Geometry check sheet. Reference: the model listing, model coordinates, mm. Face numbers are marked on the shaded views. Round coordinates to 2 decimals unless told otherwise and drop trailing zeros. Order: outer loops, then holes, each group sorted by start corner. A loop starts at its lowest first (then second) coordinate and runs counter-clockwise, first axis right, second up.
(1) Go/stop test with flat-tipped pins: pin 1 (10 mm diameter, centred on x = 27, z = -23, fed in from +Y); pin 2 (3.5 mm diameter, centred on x = 101, z = -11, fed in from -Y). Record where each tip stops, or that it passes through.
(2) Sectioned sample at C-C (z = -69). Record the boundary of the cut face in (x, y).
(3) Material ranges on line 1 along X through (y, z) = (3.5, -23); line 2 along Z through (x, y) = (-3.5, 8.05); line 3 along Z through (x, y) = (99.5, 1.3), recorded low to high.
(4) Sectioned sample at D-D (x = 70.5). Record the boundary of the cut face in (y, z).
(5) Sectioned sample at A-A (y = 3.75). Give the number of separate pieces and of enclosed holes in the cut face, plus the area to 3 significant figures.
(6) Sectioned sample at B-B (z = -53). Record the boundary of the cut face in (x, y).
(7) Release check for a two-part mould opening along X. For the marked faces 1, 2 and 3 record: +X half, -X half, draft (parallel to the pull), parting line (faces both ways), or undercut.
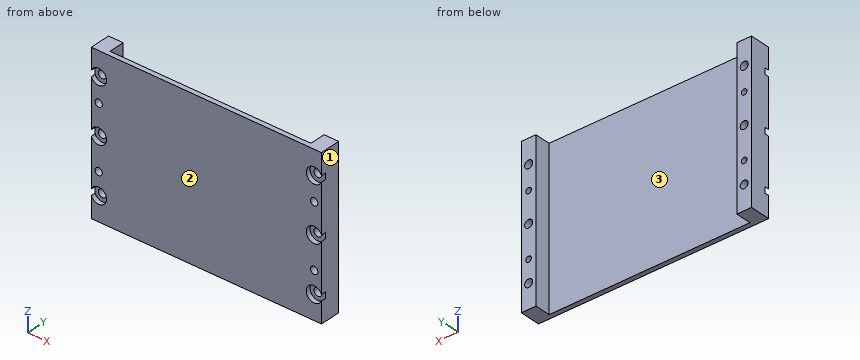
from build123d import *

# Parameters (mm, degrees)
SKETCH1_W                                      = 96
SKETCH1_H                                      = 75
BOSS_EXTRUDE1_DEPTH                            = 2.3
SKETCH2_W                                      = 7
SKETCH2_H                                      = 75
BOSS_EXTRUDE2_DEPTH                            = 7.5
BOSS_EXTRUDE2_DEPTH_BACK                       = 2.3
BOSS_EXTRUDE3_REACH                            = 9.5
SKETCH3_W                                      = 7
SKETCH3_H                                      = 75
BOSS_EXTRUDE3_DIRECTION_2_REACH                = 4.3
F_6_32_TAPPED_HOLE1_D                          = 2.7051
F_6_32_TAPPED_HOLE1_CBORE_D                    = 3.5052
F_6_32_TAPPED_HOLE1_CBORE_DEPTH                = 7.01
CBORE_FOR_6_BUTTON_HEAD_CAP_SCREW1_D           = 3.7973
CBORE_FOR_6_BUTTON_HEAD_CAP_SCREW1_CBORE_D     = 7.54126
CBORE_FOR_6_BUTTON_HEAD_CAP_SCREW1_CBORE_DEPTH = 2.1541994


with BuildPart() as part:
    # Sketch1 → Boss-Extrude1 (new body)
    with BuildSketch(Plane(origin=(0, 0, 0), x_dir=(1, 0, 0), z_dir=(0, 1, 0))):
        with Locations((48, 37.5)):
            Rectangle(SKETCH1_W, SKETCH1_H)
    extrude(amount=BOSS_EXTRUDE1_DEPTH)

    # Sketch2 → Boss-Extrude2 (add, two sides)
    with BuildSketch(Plane(origin=(0, 2.3, 0), x_dir=(1, 0, 0), z_dir=(0, 1, 0))) as boss_extrude2_sk:
        with Locations((-3.5, 37.5)):
            Rectangle(SKETCH2_W, SKETCH2_H)
    extrude(amount=BOSS_EXTRUDE2_DEPTH)
    extrude(boss_extrude2_sk.sketch, amount=-BOSS_EXTRUDE2_DEPTH_BACK)

    # Boss-Extrude3: up to this face of the body (flat: up to its plane)
    boss_extrude3_end = Plane(part.part.faces().sort_by_distance((-3.5, 9.8, -37.5))[0])
    # Sketch3 → Boss-Extrude3 (add, up to the picked face)
    with BuildSketch(Plane(origin=(0, 2.3, 0), x_dir=(1, 0, 0), z_dir=(0, 1, 0)), mode=Mode.PRIVATE) as boss_extrude3_sk1:
        with Locations((99.5, 37.5)):
            Rectangle(SKETCH3_W, SKETCH3_H)
    boss_extrude3_tool1 = split(extrude(boss_extrude3_sk1.sketch, amount=BOSS_EXTRUDE3_REACH, mode=Mode.PRIVATE), bisect_by=boss_extrude3_end, keep=Keep.BOTH, mode=Mode.PRIVATE)
    add(boss_extrude3_tool1.solids().sort_by_distance((99.5, 2.3, -37.5))[0])

    # Boss-Extrude3 direction 2: up to this face of the body (flat: up to its plane)
    boss_extrude3_direction_2_end = Plane(part.part.faces().sort_by_distance((44.5, 0, -37.5))[0])
    # Sketch3 → Boss-Extrude3 direction 2 (add, up to the picked face)
    with BuildSketch(Plane(origin=(0, 2.3, 0), x_dir=(1, 0, 0), z_dir=(0, 1, 0)), mode=Mode.PRIVATE) as boss_extrude3_direction_2_sk1:
        with Locations((99.5, 37.5)):
            Rectangle(SKETCH3_W, SKETCH3_H)
    boss_extrude3_direction_2_tool1 = split(extrude(boss_extrude3_direction_2_sk1.sketch, amount=-BOSS_EXTRUDE3_DIRECTION_2_REACH, mode=Mode.PRIVATE), bisect_by=boss_extrude3_direction_2_end, keep=Keep.BOTH, mode=Mode.PRIVATE)
    add(boss_extrude3_direction_2_tool1.solids().sort_by_distance((99.5, 2.3, -37.5))[0])

    # #6-32 Tapped Hole1 (through all)
    with Locations(Plane(origin=(0, 0, 0), x_dir=(-1, 0, 0), z_dir=(0, -1, 0))):
        with Locations((-99.5, 23), (-99.5, 53), (3.5, 23), (3.5, 53)):
            CounterBoreHole(F_6_32_TAPPED_HOLE1_D / 2, F_6_32_TAPPED_HOLE1_CBORE_D / 2, F_6_32_TAPPED_HOLE1_CBORE_DEPTH)

    # CBORE for #6 Button Head Cap Screw1 (through all)
    with Locations(Plane(origin=(0, 0, 0), x_dir=(-1, 0, 0), z_dir=(0, -1, 0))):
        with Locations((-99.5, 63.5), (-99.5, 37.5), (-99.5, 11.5), (3.5, 11.5), (3.5, 37.5), (3.5, 63.5)):
            CounterBoreHole(CBORE_FOR_6_BUTTON_HEAD_CAP_SCREW1_D / 2, CBORE_FOR_6_BUTTON_HEAD_CAP_SCREW1_CBORE_D / 2, CBORE_FOR_6_BUTTON_HEAD_CAP_SCREW1_CBORE_DEPTH)


solid = part.part
Answer below:
1. pin 1: stops at y = 2.3
1. pin 2: stops at y = 2.15
2. outline: (-7, 0) - (103, 0) - (103, 9.8) - (96, 9.8) - (96, 2.3) - (0, 2.3) - (0, 9.8) - (-7, 9.8) - close
3. line 1: x = -7 to -5.25, -1.75 to 0, 96 to 97.75, 101.25 to 103
3. line 2: z = -75 to -65.4, -61.6 to -54.35, -51.65 to -39.4, -35.6 to -24.35, -21.65 to -13.4, -9.6 to 0
3. line 3: z = -75 to -67.27, -59.73 to -54.75, -51.25 to -41.27, -33.73 to -24.75, -21.25 to -15.27, -7.73 to 0
4. outline: (0, -75) - (2.3, -75) - (2.3, 0) - (0, 0) - close
5. separate pieces: 2
5. enclosed holes: 10
5. area: 943 mm2
6. outline: (-7, 0) - (-5.25, 0) - (-5.25, 7.01) - (-4.85, 7.01) - (-4.85, 9.8) - (-7, 9.8) - close; (-2.15, 7.01) - (-1.75, 7.01) - (-1.75, 0) - (97.75, 0) - (97.75, 7.01) - (98.15, 7.01) - (98.15, 9.8) - (96, 9.8) - (96, 2.3) - (0, 2.3) - (0, 9.8) - (-2.15, 9.8) - close; (100.85, 7.01) - (101.25, 7.01) - (101.25, 0) - (103, 0) - (103, 9.8) - (100.85, 9.8) - close
7. face 1: +X half
7. face 2: draft
7. face 3: undercut
